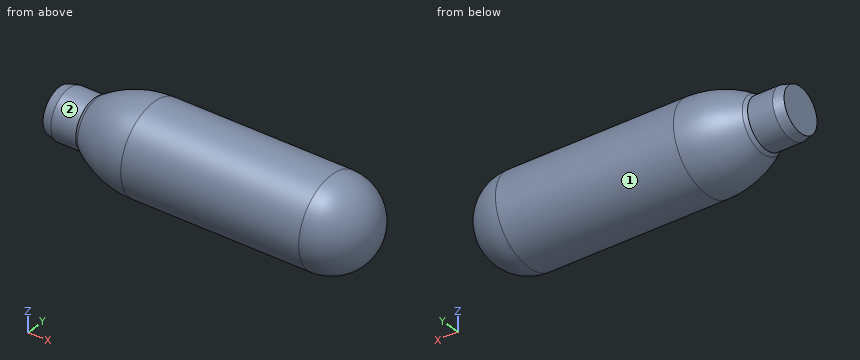
```python
from build123d import *

# Parameters (mm, degrees)
F2_R = 9


with BuildPart() as f1:
    # F0 (on Front) → F1 (revolve)
    with BuildSketch(Plane.XZ):
        with BuildLine():
            Line((-64, 0), (0, 0))
            Line((0, 0), (0, 9))
            Line((0, 9), (-44.969352, 9))
            ThreePointArc((-44.969352, 9), (-50.897358, 8.101276), (-56.292601, 5.485874))
            Line((-56.292601, 5.485874), (-57, 5))
            Line((-57, 5), (-62.063508, 5))
            Line((-62.063508, 5), (-64, 4.5))
            Line((-64, 4.5), (-64, 0))
        make_face()
    revolve(axis=Axis((-32, 0, 0), (-1, 0, 0)))

    # F2
    f2_edges = [f1.edges().sort_by_distance(p)[0] for p in [
        (0, 0, -9),
        (-44.969352, 0, -9),
        (-22.484676, 0, 9),
    ]]
    fillet(f2_edges, radius=F2_R)


solid = f1.part
```
Verification items for the finished model (mm, model axes). Face numbers are marked on the shaded views. A direction names the side the tool comes from. Give positions to 0.01 mm unless a question says otherwise; leave off trailing zeros. Order: outer loops, then holes, each group sorted by start corner. A loop starts at its lowest first (then second) coordinate and runs counter-clockwise, first axis right, second up. Notation, with made-up numbers: (57, 50) -> (78, 50) arc R19 ccw to (78, 75) -> close; hole circle Ø4 at (55, -5.75). An arc over 180 degrees is marked (long way). One line per item, written item: value.
(1) Gauge pin test, flat ends, axial feed: pin 1 (3 mm diameter, centred on y = -3.5, z = 0.5, fed in from +X); pin 2 (4 mm diameter, centred on x = -38, z = -3, fed in from -Y). Record the tip position at first contact, or that the pin passes through.
Final values:
pin 1: x = -0.23
pin 2: y = -8.94
(2) Sectioned sample at A-A on x = -58. Record the cut outline in (y, z), then the cut area to 3 significant figures.
Final values:
outline: circle Ø10 at (0, 0)
area: 78.5 mm^2
(3) Scan lines: line 1 along Z through (x, y) = (-57, -0.75); line 2 along Y through (x, z) = (-17, 6); line 3 along X through (y, z) = (5, 3.25). Record each from-to range of solid material in increasing order. Write a range as [from, to].
Final values:
line 1: [-4.94, 4.94]
line 2: [-6.71, 6.71]
line 3: [-55.56, -2.26]
(4) Tool access check on the marked faces 1 and 2. Record the directions out of +Z, -Z, +X, -X, +Y, -Y that give a thin tool (end or side, any length) a straight path to the whole face; none if there is none.
Final values:
face 1: +X, -X
face 2: -X
(5) Sectioned sample at B-B on x = -21.5. Record the cut outline in (y, z).
Final values:
outline: circle Ø18 at (0, 0)
